The figure shows three views and two pictorial views of one solid part (mm, origin at its lowest corner). Answer the questions. Round coordinates to 2 decimals unless told otherwise and drop trailing zeros. Loops run counter-clockwise (first coordinate to the right, second up) from the corner with the lowest first, then second, coordinate; pieces in that order, holes last. Notation, with made-up numbers: (0, -13.5) -> (8, -13.5) arc R23 ccw to (8, 17.5) -> close; hole circle Ø3 at (-5, 15.25). An arc over 180 degrees is marked (long way). Put each result on its own line as item: value.
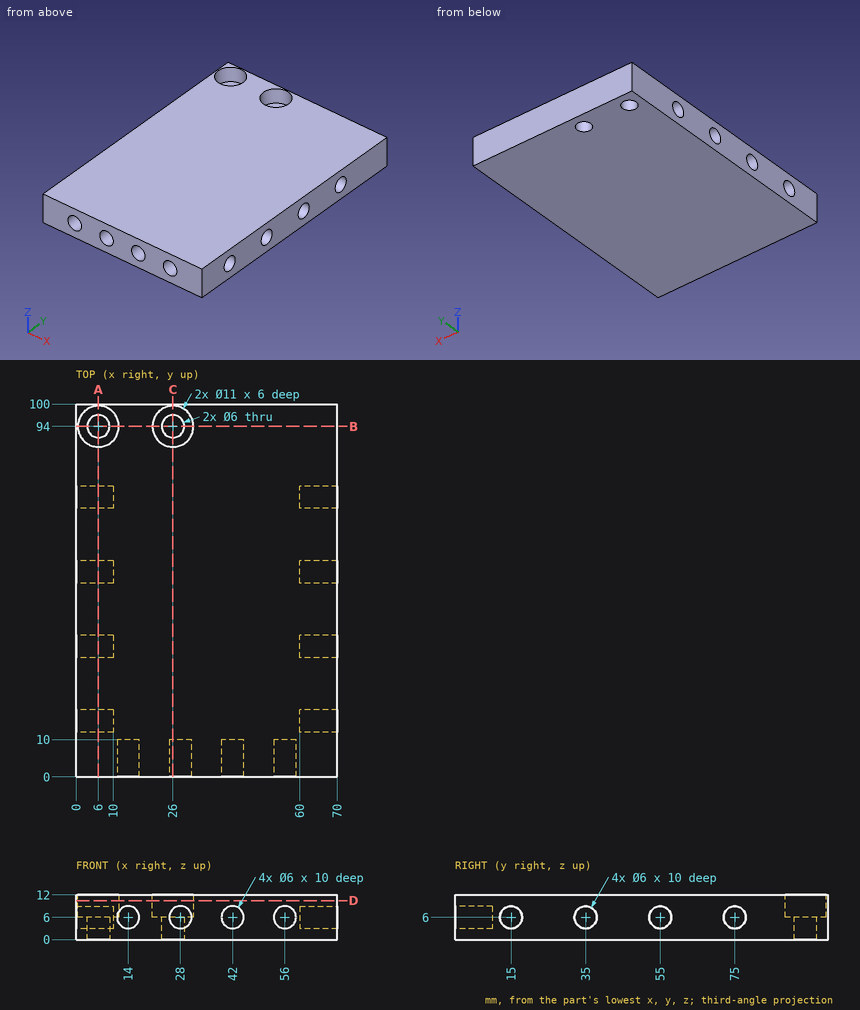
Item 1: The part is cut by section C-C (x = 26). Determine the outline of the cut face in (y, z).
Derived:
outline: (0, 0) -> (91, 0) -> (91, 6) -> (88.5, 6) -> (88.5, 12) -> (0, 12) -> (0, 8.24) -> (10, 8.24) -> (10, 3.76) -> (0, 3.76) -> close; (97, 0) -> (100, 0) -> (100, 12) -> (99.5, 12) -> (99.5, 6) -> (97, 6) -> close
Item 2: The part is cut by section A-A (x = 6). Determine the outline of the cut face in (y, z), then the cut area to 3 significant figures.
Derived:
outline: (0, 0) -> (91, 0) -> (91, 6) -> (88.5, 6) -> (88.5, 12) -> (0, 12) -> close; (97, 0) -> (100, 0) -> (100, 12) -> (99.5, 12) -> (99.5, 6) -> (97, 6) -> close; hole circle Ø6 at (15, 6); hole circle Ø6 at (35, 6); hole circle Ø6 at (55, 6); hole circle Ø6 at (75, 6)
area: 985 mm^2
Item 3: Flat-ended cylindrical pins translate along their axes: pin 1 Ø3 at (y, z) = (14, 6) entering from -X; pin 2 Ø5 at (y, z) = (15, 6) entering from +X; pin 3 Ø3.5 at (x, y) = (26, 94) entering from -Z; pin 4 Ø5.5 at (x, y) = (26, 96.5) entering from +Z. Find the tip coordinate at first contact, or state that the pin passes through.
Derived:
pin 1: stops at x = 10
pin 2: stops at x = 60
pin 3: passes through
pin 4: stops at z = 6
Item 4: The part is cut by section D-D (z = 10.5). Determine the outline of the cut face in (x, y).
Derived:
outline: (0, 0) -> (70, 0) -> (70, 100) -> (0, 100) -> close; hole circle Ø11 at (6, 94); hole circle Ø11 at (26, 94)
Item 5: The part is cut by section B-B (y = 94). Determine the outline of the cut face in (x, z).
Derived:
outline: (0, 0) -> (3, 0) -> (3, 6) -> (0.5, 6) -> (0.5, 12) -> (0, 12) -> close; (9, 0) -> (23, 0) -> (23, 6) -> (20.5, 6) -> (20.5, 12) -> (11.5, 12) -> (11.5, 6) -> (9, 6) -> close; (29, 0) -> (70, 0) -> (70, 12) -> (31.5, 12) -> (31.5, 6) -> (29, 6) -> close
Item 6: Find the intervals of material crossed by line 1 along Y through (x, z) = (66.75, 6); line 2 along Z through (x, y) = (14, 7); line 3 along Y through (x, z) = (26, 9.15), in increasing order.
Derived:
line 1: y = 0 to 12, 18 to 32, 38 to 52, 58 to 72, 78 to 100
line 2: z = 0 to 3, 9 to 12
line 3: y = 0 to 88.5, 99.5 to 100
